Here's how the part is built. I have some questions about the finished solid (model axes, mm). Face numbers are marked on the shaded views. Coordinates: 2 decimals unless noted, no trailing zeros. Order: outer loops, then holes, each group sorted by start corner. A loop starts at its lowest first (then second) coordinate and runs counter-clockwise, first axis right, second up. Notation, with made-up numbers: (-2.75, -40) -> (18.25, -40) arc R17 cw to (18.25, -13) -> close; hole circle Ø1 at (48.25, 63). An arc over 180 degrees is marked (long way). One line per item, written item: value. Start each with the question number.
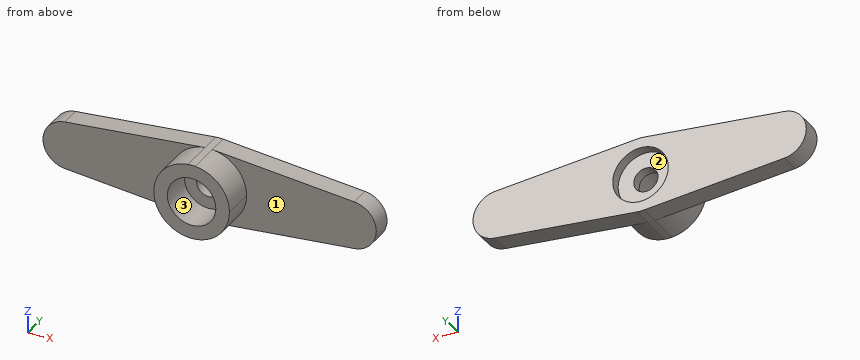
```python
from build123d import *
from build123d.topology import SkipClean

# Parameters (mm, degrees)
SKETCH1_R           = 1.2
BOSS_EXTRUDE1_DEPTH = 2
BOSS_EXTRUDE2_START = 3.2
SKETCH2_R           = 1.2
BOSS_EXTRUDE2_DEPTH = 3.2
SKETCH3_R           = 2.4
CUT_EXTRUDE3_DEPTH  = 3.2
SKETCH4_R           = 2.75
CUT_EXTRUDE4_DEPTH  = 1


with BuildPart() as part:
    # Sketch1 → Boss-Extrude1 (new body)
    with BuildSketch(Plane(origin=(0, 0, 0), x_dir=(1, 0, 0), z_dir=(0, 1, 0))):
        with BuildLine():
            Line((0.356514085, 3.73301456), (14.428169014, 2.389129319))
            ThreePointArc((14.428169014, 2.389129319), (16.6, 0), (14.428169014, -2.389129319))
            Line((14.428169014, -2.389129319), (0.356514085, -3.73301456))
            ThreePointArc((0.356514085, -3.73301456), (-0.00225279, -3.749999323), (-0.360998998, -3.732583519))
            Line((-0.360998998, -3.732583519), (-14.254623989, -2.388853452))
            ThreePointArc((-14.254623989, -2.388853452), (-16.42358463, 0), (-14.254623989, 2.388853452))
            Line((-14.254623989, 2.388853452), (-0.360998998, 3.732583519))
            ThreePointArc((-0.360998998, 3.732583519), (-0.00225279, 3.749999323), (0.356514085, 3.73301456))
        make_face()
        with Locations(Location((0, 0, 0), (0, 0, 270))):
            Circle(SKETCH1_R, mode=Mode.SUBTRACT)
    extrude(amount=BOSS_EXTRUDE1_DEPTH)

    # Sketch2 → Boss-Extrude2 (add)
    with SkipClean():  # the faces are left unmerged after this step: merging them gives an invalid solid
        with BuildSketch(Plane.XZ.offset(BOSS_EXTRUDE2_START)):
            with BuildLine():
                ThreePointArc((3.75, 0), (2.774835835, 2.522456361), (0.356514085, 3.73301456))
                ThreePointArc((0.356514085, 3.73301456), (-0.00225279, 3.749999323), (-0.360998998, 3.732583519))
                ThreePointArc((-0.360998998, 3.732583519), (-3.75, 0), (-0.360998998, -3.732583519))
                ThreePointArc((-0.360998998, -3.732583519), (-0.00225279, -3.749999323), (0.356514085, -3.73301456))
                ThreePointArc((0.356514085, -3.73301456), (2.774835835, -2.522456361), (3.75, 0))
            make_face()
            with Locations(Location((0, 0, 0), (0, 0, 270))):
                Circle(SKETCH2_R, mode=Mode.SUBTRACT)
        extrude(amount=-BOSS_EXTRUDE2_DEPTH)

    # Sketch3 → Cut-Extrude3 (cut)
    with BuildSketch(Plane.XZ.offset(3.2)):
        with Locations(Location((0, 0, 0), (0, 0, 270))):
            Circle(SKETCH3_R)
    extrude(amount=-CUT_EXTRUDE3_DEPTH, mode=Mode.SUBTRACT)

    # Sketch4 → Cut-Extrude4 (cut)
    with BuildSketch(Plane(origin=(0, 2, 0), x_dir=(1, 0, 0), z_dir=(0, 1, 0))):
        with Locations(Location((0, 0, 0), (0, 0, 270))):
            Circle(SKETCH4_R)
    extrude(amount=-CUT_EXTRUDE4_DEPTH, mode=Mode.SUBTRACT)


solid = part.part
```
Q1. Imagine slicing it at C-C (z = 0.75). Write out the boundary of the cut face in (x, y).
Q2. If we mould it in two halves opening along Z, with no side actions, what happens to the marked faces 1, 2 and 3? For each: +Z half, -Z half, draft (parallel to the pull), parting line (faces both ways), or undercut.
Q3. For P1, Ø3, axis at x = 7.5, z = -2.5, coming from the -Y side; P2, Ø2, axis at y = 0.5, z = -0.5, coming from the -X side; P3, Ø3, axis at x = 0, z = 0, coming from the +Y side, each with a flat end and sliding along its axis, tell me the tip position at first contact or that it passes through.
Q4. Imagine slicing it at B-B (x = 0). Write out the boundary of the cut face in (y, z), plus the area to 3 significant figures.
Q5. Imagine slicing it at A-A (y = -2.45). Write out the boundary of the cut face in (x, z), plus the area to 3 significant figures.
Q6. Imagine slicing it at D-D (y = 0.45). Write out the boundary of the cut face in (x, z), plus the area to 3 significant figures.
Q7. I need wall thicknesses on line 1 (Y direction, x = 5, z = -0.5); line 2 (X direction, y = 1.55, z = 0); line 3 (Z direction, x = 0, y = 0.8). Which ranges of each line are inside material? Lowest first, please.
Completed:
1. outline: (-16.3, 0) -> (-3.67, 0) -> (-3.67, -3.2) -> (-2.28, -3.2) -> (-2.28, 0) -> (-0.94, 0) -> (-0.94, 1) -> (-2.65, 1) -> (-2.65, 2) -> (-16.3, 2) -> close; (0.94, 0) -> (2.28, 0) -> (2.28, -3.2) -> (3.67, -3.2) -> (3.67, 0) -> (16.48, 0) -> (16.48, 2) -> (2.65, 2) -> (2.65, 1) -> (0.94, 1) -> close
2. face 1: draft
2. face 2: undercut
2. face 3: undercut
3. P1: stops at y = 0
3. P2: stops at x = -16.42
3. P3: stops at y = 1
4. outline: (-3.2, -3.75) -> (2, -3.75) -> (2, -2.75) -> (1, -2.75) -> (1, -1.2) -> (0, -1.2) -> (0, -2.4) -> (-3.2, -2.4) -> close; (-3.2, 2.4) -> (0, 2.4) -> (0, 1.2) -> (1, 1.2) -> (1, 2.75) -> (2, 2.75) -> (2, 3.75) -> (-3.2, 3.75) -> close
4. area: 15.7 mm2
5. outline: circle Ø7.5 at (0, 0); hole circle Ø4.8 at (0, 0)
5. area: 26.1 mm2
6. outline: (-14.25, -2.39) -> (-0.36, -3.73) arc R3.75 ccw to (0.36, -3.73) -> (14.43, -2.39) arc R2.4 ccw to (14.43, 2.39) -> (0.36, 3.73) arc R3.75 ccw to (-0.36, 3.73) -> (-14.25, 2.39) arc R2.4 ccw to start; hole circle Ø2.4 at (0, 0)
6. area: 188 mm2
7. line 1: y = 0 to 2
7. line 2: x = -16.42 to -2.75, 2.75 to 16.6
7. line 3: z = -3.75 to -1.2, 1.2 to 3.75
